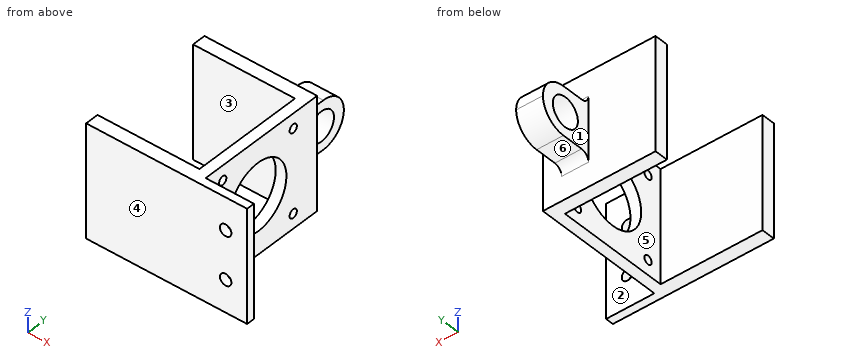
from build123d import *

# Parameters (mm, degrees)
SKETCH1_W            = 94
SKETCH1_H            = 42
BOSS_EXTRUDE1_DEPTH  = 3
SKETCH2_W            = 4
SKETCH2_H            = 42
BOSS_EXTRUDE2_DEPTH  = 47
SKETCH3_R            = 12.5
SKETCH3_R_2          = 1.6
CUT_EXTRUDE1_DEPTH   = 114.176852757
SKETCH4_W            = 42
SKETCH4_H            = 5
BOSS_EXTRUDE3_DEPTH  = 40
SKETCH5_W            = 42
SKETCH5_H            = 5
BOSS_EXTRUDE4_DEPTH  = 38
SKETCH7_W            = 42
SKETCH7_H            = 42
SKETCH7_W_2          = 44
BOSS_EXTRUDE6_DEPTH  = 5
SKETCH9_R            = 2.15
CUT_EXTRUDE2_DEPTH   = 149.731301346
SKETCH11_W           = 10
SKETCH11_H           = 18
BOSS_EXTRUDE7_DEPTH  = 20
SKETCH13_R           = 5.5
CUT_EXTRUDE3_DEPTH   = 169.988165266
BOSS_EXTRUDE11_DEPTH = 5
SKETCH23_W           = 10
SKETCH23_H           = 26
BOSS_EXTRUDE12_DEPTH = 50
CUT_EXTRUDE7_DEPTH   = 193.595430891
SKETCH25_W           = 10
SKETCH25_H           = 18
BOSS_EXTRUDE13_DEPTH = 20
SKETCH26_R           = 5.5
CUT_EXTRUDE8_DEPTH   = 193.595430891
SKETCH27_W           = 12
SKETCH27_H           = 18
BOSS_EXTRUDE14_DEPTH = 69
CUT_EXTRUDE10_START  = -5
SKETCH28_R           = 5.5
CUT_EXTRUDE10_DEPTH  = 5
SKETCH29_R           = 5.5
CUT_EXTRUDE11_DEPTH  = 5
FILLET4_R            = 9
FILLET3_R            = 3
SKETCH30_W           = 112
SKETCH30_H           = 120
CUT_EXTRUDE13_DEPTH  = 181.413414135


# Some blends are built 0.0001 mm under size
with BuildPart() as part:
    # Sketch1 → Boss-Extrude1 (new body)
    with BuildSketch(Plane(origin=(0, 0, 0), x_dir=(1, 0, 0), z_dir=(0, 1, 0))):
        with Locations((47, -21)):
            Rectangle(SKETCH1_W, SKETCH1_H)
    extrude(amount=BOSS_EXTRUDE1_DEPTH)

    # Sketch2 → Boss-Extrude2 (add)
    with BuildSketch(Plane.XZ):
        with Locations((2, 21)):
            Rectangle(SKETCH2_W, SKETCH2_H)
        with Locations((92, 21)):
            Rectangle(SKETCH2_W, SKETCH2_H)
    extrude(amount=-BOSS_EXTRUDE2_DEPTH)

    # Sketch3 → Cut-Extrude1 (cut, through all)
    with BuildSketch(Plane(origin=(94, 0, 0), x_dir=(0, 0, -1), z_dir=(1, 0, 0))):
        with Locations((-21, 26)):
            Circle(SKETCH3_R)
        with Locations((-36.5, 41.5)):
            Circle(SKETCH3_R_2)
        with Locations((-5.5, 41.5)):
            Circle(SKETCH3_R_2)
        with Locations((-36.5, 10.5)):
            Circle(SKETCH3_R_2)
        with Locations((-5.5, 10.5)):
            Circle(SKETCH3_R_2)
    extrude(amount=-CUT_EXTRUDE1_DEPTH, mode=Mode.SUBTRACT)

    # Sketch4 → Boss-Extrude3 (add)
    with BuildSketch(Plane(origin=(94, 0, 0), x_dir=(0, 0, -1), z_dir=(1, 0, 0))):
        with Locations((-21, 2.5)):
            Rectangle(SKETCH4_W, SKETCH4_H)
    extrude(amount=BOSS_EXTRUDE3_DEPTH)

    # Sketch5 → Boss-Extrude4 (add)
    with BuildSketch(Plane.ZY):
        with Locations((21, 2.5)):
            Rectangle(SKETCH5_W, SKETCH5_H)
    extrude(amount=BOSS_EXTRUDE4_DEPTH)

    # Sketch7 → Boss-Extrude6 (add)
    with BuildSketch(Plane(origin=(0, 47, 0), x_dir=(1, 0, 0), z_dir=(0, 1, 0))):
        with Locations((-17, -21)):
            Rectangle(SKETCH7_W, SKETCH7_H)
        with Locations((112, -21)):
            Rectangle(SKETCH7_W_2, SKETCH7_H)
    extrude(amount=BOSS_EXTRUDE6_DEPTH)

    # Sketch9 → Cut-Extrude2 (cut, through all)
    with BuildSketch(Plane(origin=(0, 3, 0), x_dir=(1, 0, 0), z_dir=(0, 1, 0))):
        with Locations(Location((83, -20, 0), (0, 0, 270))):
            Circle(SKETCH9_R)
        with Locations(Location((65, -20, 0), (0, 0, 270))):
            Circle(SKETCH9_R)
        with Locations(Location((74, -11, 0), (0, 0, 270))):
            Circle(SKETCH9_R)
        with Locations(Location((74, -29, 0), (0, 0, 270))):
            Circle(SKETCH9_R)
        with Locations(Location((14, -12, 0), (0, 0, 270))):
            Circle(SKETCH9_R)
        with Locations(Location((14, -30, 0), (0, 0, 270))):
            Circle(SKETCH9_R)
        with Locations(Location((30, -12, 0), (0, 0, 270))):
            Circle(SKETCH9_R)
        with Locations(Location((30, -30, 0), (0, 0, 270))):
            Circle(SKETCH9_R)
    extrude(amount=-CUT_EXTRUDE2_DEPTH, mode=Mode.SUBTRACT)

    # Sketch11 → Boss-Extrude7 (add)
    with BuildSketch(Plane(origin=(0, 52, 0), x_dir=(1, 0, 0), z_dir=(0, 1, 0))):
        with Locations((-8, -21)):
            Rectangle(SKETCH11_W, SKETCH11_H)
        with Locations((107, -21)):
            Rectangle(SKETCH11_W, SKETCH11_H)
    extrude(amount=BOSS_EXTRUDE7_DEPTH)

    # Sketch13 → Cut-Extrude3 (cut, through all)
    with BuildSketch(Plane.ZY.offset(13)):
        with Locations((21, 62.15)):
            Circle(SKETCH13_R)
    extrude(amount=-CUT_EXTRUDE3_DEPTH, mode=Mode.SUBTRACT)

    # Sketch20 → Boss-Extrude11 (add)
    with BuildSketch(Plane.XY.offset(42)):
        Polygon((134, 0), (134, 52), (90, 52), (90, 0), (95, 0), (95, 20), (102, 26), (112, 26), (129, 20), (129, 0), align=None)
    extrude(amount=BOSS_EXTRUDE11_DEPTH)

    # Sketch23 → Boss-Extrude12 (add)
    with BuildSketch(Plane.XY.offset(47)):
        with Locations((107, 39)):
            Rectangle(SKETCH23_W, SKETCH23_H)
    extrude(amount=BOSS_EXTRUDE12_DEPTH)

    # Sketch24 → Cut-Extrude7 (cut, through all)
    with BuildSketch(Plane(origin=(112, 0, 0), x_dir=(0, 0, -1), z_dir=(1, 0, 0))):
        Polygon((-47, 26), (-97, 39), (-97, 26), align=None)
    extrude(amount=-CUT_EXTRUDE7_DEPTH, mode=Mode.SUBTRACT)

    # Sketch25 → Boss-Extrude13 (add)
    with BuildSketch(Plane(origin=(0, 52, 0), x_dir=(1, 0, 0), z_dir=(0, 1, 0))):
        with Locations((107, -71)):
            Rectangle(SKETCH25_W, SKETCH25_H)
    extrude(amount=BOSS_EXTRUDE13_DEPTH)

    # Sketch26 → Cut-Extrude8 (cut, through all)
    with BuildSketch(Plane(origin=(112, 0, 0), x_dir=(0, 0, -1), z_dir=(1, 0, 0))):
        with Locations((-71, 62.15)):
            Circle(SKETCH26_R)
    extrude(amount=-CUT_EXTRUDE8_DEPTH, mode=Mode.SUBTRACT)

    # Sketch27 → Boss-Extrude14 (add)
    with BuildSketch(Plane(origin=(0, 3, 0), x_dir=(1, 0, 0), z_dir=(0, 1, 0))):
        with Locations((47, -21)):
            Rectangle(SKETCH27_W, SKETCH27_H)
    extrude(amount=BOSS_EXTRUDE14_DEPTH)

    # Sketch28 → Cut-Extrude10 (cut)
    with BuildSketch(Plane(origin=(53, 0, 0), x_dir=(0, 0, -1), z_dir=(1, 0, 0)).offset(CUT_EXTRUDE10_START)):
        with Locations(Location((-21, 62.15, 0), (0, 0, 180))):
            Circle(SKETCH28_R)
    extrude(amount=CUT_EXTRUDE10_DEPTH, mode=Mode.SUBTRACT)

    # Sketch29 → Cut-Extrude11 (cut)
    with BuildSketch(Plane.ZY.offset(-41)):
        with Locations((21, 62.15)):
            Circle(SKETCH29_R)
    extrude(amount=-CUT_EXTRUDE11_DEPTH, mode=Mode.SUBTRACT)

    # Fillet4
    fillet4_edges = [part.edges().sort_by_distance(p)[0] for p in [
        (-8, 72, 12),
        (-8, 72, 30),
        (107, 72, 12),
        (107, 72, 30),
        (107, 72, 62),
        (107, 72, 80),
        (47, 72, 12),
        (47, 72, 30),
    ]]
    fillet(fillet4_edges, radius=FILLET4_R - 0.0001)  # a hair under: the kernel refuses the full size

    # Fillet3
    # the kernel refuses this fillet: 3 mm, written as the material it adds along each edge
    with BuildSketch(Plane(origin=(-3, 52, 30), x_dir=(0, 1, 0), z_dir=(-1, 0, 0)), Plane(origin=(112, 52, 80), x_dir=(0, 1, 0), z_dir=(-1, 0, 0))) as fillet3_piece_1:
        with BuildLine():
            CenterArc((FILLET3_R, -FILLET3_R), FILLET3_R, 90, 90)
            Line((0, -FILLET3_R), (0, 0))
            Line((0, 0), (FILLET3_R, 0))
        make_face()
    extrude(amount=10)
    with BuildSketch(Plane(origin=(-13, 52, 12), x_dir=(0, 0, -1), z_dir=(1, 0, 0)), Plane(origin=(112, 52, 30), x_dir=(0, 0, 1), z_dir=(-1, 0, 0)), Plane(origin=(102, 52, 12), x_dir=(0, 0, -1), z_dir=(1, 0, 0)), Plane(origin=(102, 52, 62), x_dir=(0, 0, -1), z_dir=(1, 0, 0))) as fillet3_piece_2:
        with BuildLine():
            CenterArc((FILLET3_R, FILLET3_R), FILLET3_R, 180, 90)
            Line((0, FILLET3_R), (0, 0))
            Line((0, 0), (FILLET3_R, 0))
        make_face()
    extrude(amount=10)
    with BuildSketch(Plane(origin=(95, 20, 42), x_dir=(0, -1, 0), z_dir=(0, 0, 1))) as fillet3_piece_3:
        with BuildLine():
            CenterArc((FILLET3_R * 0.45993492247, FILLET3_R), FILLET3_R, 220.601294645, 49.398705355)
            Line((-FILLET3_R * 0.299321679895, FILLET3_R * 0.349208626544), (0, 0))
            Line((0, 0), (FILLET3_R * 0.45993492247, 0))
        make_face()
    extrude(amount=5)
    with BuildSketch(Plane(origin=(102, 26, 42), x_dir=(-0.7592566023652966, -0.6507913734559685, 0), z_dir=(0, 0, 1))) as fillet3_piece_4:
        with BuildLine():
            CenterArc((FILLET3_R * 0.369924076215, FILLET3_R), FILLET3_R, 229.398705355, 40.601294645)
            Line((-FILLET3_R * 0.28086729724, FILLET3_R * 0.240743397635), (0, 0))
            Line((0, 0), (FILLET3_R * 0.369924076215, 0))
        make_face()
    extrude(amount=5)
    with BuildSketch(Plane(origin=(112, 26, 42), x_dir=(0.942990333582889, -0.3328201177351389, 0), z_dir=(0, 0, 1))) as fillet3_piece_5:
        with BuildLine():
            CenterArc((FILLET3_R * 0.171292729553, -FILLET3_R), FILLET3_R, 90, 19.440034828)
            Line((-FILLET3_R * 0.161527388182, -FILLET3_R * 0.0570096664171), (0, 0))
            Line((0, 0), (FILLET3_R * 0.171292729553, 0))
        make_face()
    extrude(amount=5)
    with BuildSketch(Plane(origin=(129, 20, 42), x_dir=(0, -1, 0), z_dir=(0, 0, 1))) as fillet3_piece_6:
        with BuildLine():
            CenterArc((FILLET3_R * 0.707515081019, -FILLET3_R), FILLET3_R, 90, 70.559965172)
            Line((-FILLET3_R * 0.235475252564, -FILLET3_R * 0.667179882265), (0, 0))
            Line((0, 0), (FILLET3_R * 0.707515081019, 0))
        make_face()
    extrude(amount=5)
    with BuildSketch(Plane(origin=(53, 3, 30), x_dir=(0, 0, 1), z_dir=(-1, 0, 0)), Plane(origin=(41, 3, 12), x_dir=(0, 0, -1), z_dir=(1, 0, 0))) as fillet3_piece_7:
        with BuildLine():
            CenterArc((FILLET3_R, FILLET3_R), FILLET3_R, 180, 90)
            Line((0, FILLET3_R), (0, 0))
            Line((0, 0), (FILLET3_R, 0))
        make_face()
    extrude(amount=12)
    # the kernel refuses this fillet: 3 mm, written as the material it takes off along each edge
    with BuildSketch(Plane(origin=(94.5, 52, 97), x_dir=(0, 0, -1), z_dir=(1, 0, 0))) as fillet3_2_piece_1:
        with BuildLine():
            CenterArc((FILLET3_R, -FILLET3_R), FILLET3_R, 90, 90)
            Line((0, -FILLET3_R), (0, 0))
            Line((0, 0), (FILLET3_R, 0))
        make_face()
    extrude(amount=25, mode=Mode.SUBTRACT)
    with BuildSketch(Plane(origin=(117.799354812, 39, 97), x_dir=(0, -0.25163385176495195, -0.9678225067882716), z_dir=(-1, 0, 0))) as fillet3_2_piece_2:
        with BuildLine():
            CenterArc((FILLET3_R * 0.773247308247, -FILLET3_R), FILLET3_R, 90, 75.425783802)
            Line((-FILLET3_R * 0.194575198541, -FILLET3_R * 0.748366148235), (0, 0))
            Line((0, 0), (FILLET3_R * 0.773247308247, 0))
        make_face()
    extrude(amount=21.598709624, mode=Mode.SUBTRACT)

    # Sketch30 → Cut-Extrude13 (cut, through all)
    with BuildSketch(Plane.XZ):
        with Locations((78, 60)):
            Rectangle(SKETCH30_W, SKETCH30_H)
    extrude(amount=-CUT_EXTRUDE13_DEPTH, mode=Mode.SUBTRACT)


solid = part.part
Could you check a few things on this model? Use its own coordinates, in mm. Face numbers are marked on the shaded views. A direction names the side the tool comes from. Round coordinates to 2 decimals unless told otherwise and drop trailing zeros. Order: outer loops, then holes, each group sorted by start corner. A loop starts at its lowest first (then second) coordinate and runs counter-clockwise, first axis right, second up.
(1) Imagine slicing it at C-C (y = 26). Write out the boundary of the cut face in (x, z).
Response values:
outline: (0, 0) - (4, 0) - (4, 8.5) - (0, 8.5) - close; (0, 33.5) - (4, 33.5) - (4, 42) - (0, 42) - close
(2) Imagine slicing it at B-B (x = -11). Count the separate pieces of the cut face and the enclosed holes in it, plus the area to 3 significant figures.
Response values:
separate pieces: 2
enclosed holes: 1
area: 654 mm2
(3) Imagine slicing it at A-A (x = 14). Write out the boundary of the cut face in (y, z), plus the area to 3 significant figures.
Response values:
outline: (0, 0) - (3, 0) - (3, 9.85) - (0, 9.85) - close; (0, 14.15) - (3, 14.15) - (3, 27.85) - (0, 27.85) - close; (0, 32.15) - (3, 32.15) - (3, 42) - (0, 42) - close
area: 100 mm2
(4) Please list where these lines run through material, in increasing order: line 1 along Y through (x, z) = (1.05, 5.5); line 2 along Y through (x, z) = (-31.5, 14); line 3 along X through (y, z) = (1.5, 12).
Response values:
line 1: y = 0 to 8.9, 12.1 to 39.9, 43.1 to 52
line 2: y = 0 to 5, 47 to 52
line 3: x = -38 to 11.85, 16.15 to 22
(5) Which directions (+Z, -Z, +X, -X, +Y, -Y) give clear straight access to the entire face, cutting with the end or side of a thin tool? Please do the marked faces 1, 2 and 3.
Response values:
face 1: +Z, -Z, -X, +Y
face 2: +Z, -Z, +X, +Y
face 3: +Z, -Z, -X
(6) I'm going to push flat-ended pins straight in: pin 1 (10 mm diameter, centred on y = 32.5, z = 16, fed in from +X); pin 2 (4 mm diameter, centred on x = 14, z = 30, fed in from +Y); pin 3 (21 mm diameter, centred on y = 21, z = 26.5, fed in from -X); pin 4 (12 mm diameter, centred on x = -1.5, z = 13, fed in from +Y). Where does each tip first touch, or does it pass through?
Response values:
pin 1: stops at x = 4
pin 2: passes through
pin 3: stops at x = 0
pin 4: stops at y = 71.73
(7) If we mould it in two halves opening along Y, with no side actions, what happens to the marked faces 4, 5 and 6? For each: released by +Y, released by -Y, zero draft, split by the parting line, or undercut.
Response values:
face 4: released by -Y
face 5: undercut
face 6: zero draft
(8) Imagine slicing it at D-D (z = 36.5). Write out the boundary of the cut face in (x, y).
Response values:
outline: (-38, 0) - (22, 0) - (22, 3) - (4, 3) - (4, 8.9) - (0, 8.9) - (0, 5) - (-38, 5) - close; (-38, 47) - (0, 47) - (0, 43.1) - (4, 43.1) - (4, 52) - (-38, 52) - close; (0, 12.1) - (4, 12.1) - (4, 39.9) - (0, 39.9) - close
